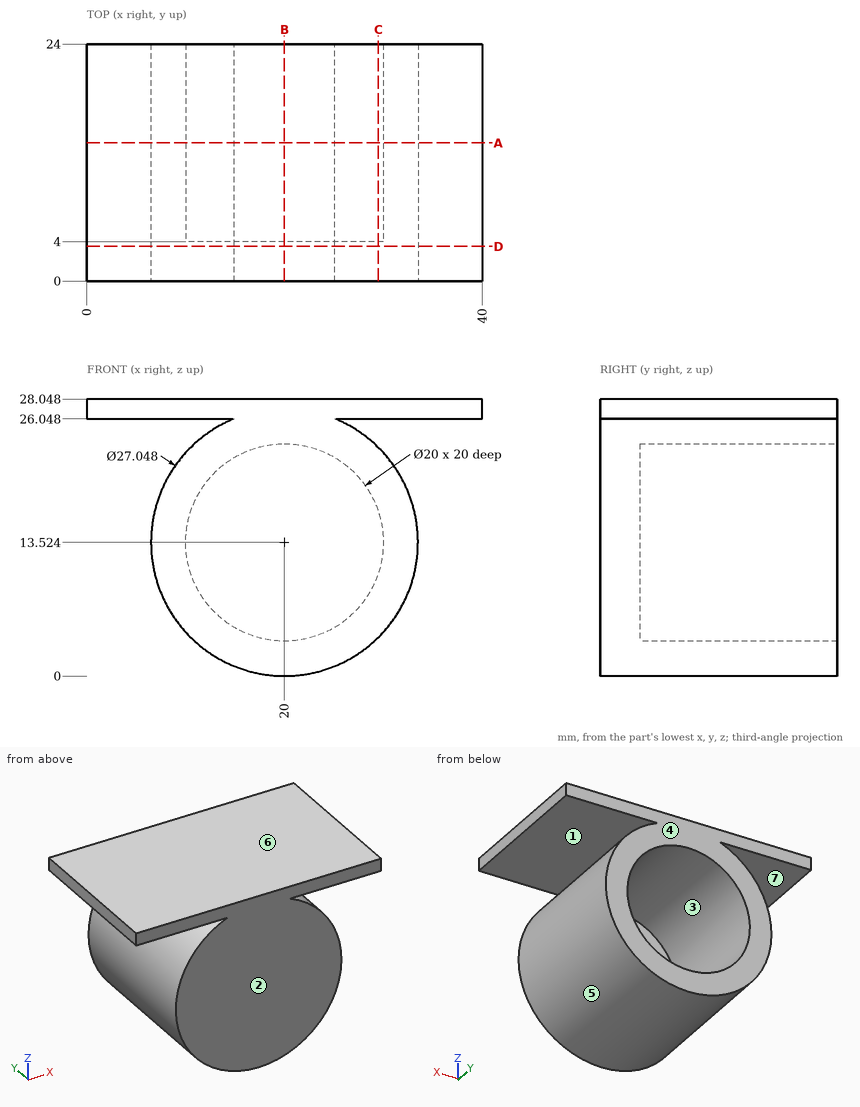
Geometry: see drawing. Coordinates: mm, zero at the bounding-box minimum. A direction names the side the tool comes from. Coordinates: 2 decimals unless noted, no trailing zeros. Loops run counter-clockwise (first coordinate to the right, second up) from the corner with the lowest first, then second, coordinate; pieces in that order, holes last. Notation, with made-up numbers: M 62,13 L 108,13 A8 ccw 108,20 Z; hole C 18.5,-20.5 d5. An arc over 180 degrees is marked long. Put each result on its own line as item: value. Start each with the question number.
1) Cut plane A-A on y = 14. Return the cut outline in (x, z), then the cut area to 3 significant figures.
2) Pull-direction query (Z, two-part tool) for the marked faces 4, 5, 6 and 7; classes: pulls with the +Z half, pulls with the -Z half, needs draft (parallel to the pull), parting line crosses it, or undercut.
3) Cut plane D-D on y = 3.5. Return the cut outline in (x, z), then the cut area to 3 significant figures.
4) Contact query for flat-ended pins moving along their axis: pin 1 Ø4 at (y, z) = (2.5, 7) entering from +X (3 decimals); pin 2 Ø4.5 at (x, y) = (11, 7) entering from -Z (3 decimals); pin 3 Ø6 at (x, y) = (7.5, 10) entering from -Z. Output: stop coordinate, or through.
5) Cut plane C-C on x = 29.5. Return the cut outline in (y, z).
6) Ray query, L1, parallel to Z at x = 29, y = 16.25 (1 decimal); L2, parallel to X at y = 12.25, z = 18.5 (1 decimal); L3, parallel to X at y = 6.25, z = 15.5. Return the intervals inside material, ascending. Write a range as from..to.
7) Cut plane B-B on x = 20. Return the cut outline in (y, z).
8) Reachability of the marked faces 1, 2 and 3 from +Z, -Z, +X, -X, +Y, -Y: full face, straight path, thin tool, end or side. Return the list, or none.
The answers:
1. outline: M 0,26.05 L 14.9,26.05 A13.52 ccw long 25.1,26.05 L 40,26.05 L 40,28.05 L 0,28.05 Z; hole C 20,13.52 d20
1. area: 334 mm²
2. face 4: needs draft
2. face 5: undercut
2. face 6: pulls with the +Z half
2. face 7: undercut
3. outline: M 0,26.05 L 14.9,26.05 A13.52 ccw long 25.1,26.05 L 40,26.05 L 40,28.05 L 0,28.05 Z
3. area: 648 mm²
4. pin 1: stops at x = 32.745
4. pin 2: stops at z = 1.805
4. pin 3: stops at z = 3.9
5. outline: M 0,3.9 L 24,3.9 L 24,10.4 L 4,10.4 L 4,16.65 L 24,16.65 L 24,23.15 L 0,23.15 Z; M 0,26.05 L 24,26.05 L 24,28.05 L 0,28.05 Z
6. L1: z = 3.4..9.2, 17.9..23.6, 26..28
6. L2: x = 7.4..11.3, 28.7..32.6
6. L3: x = 6.62..10.2, 29.8..33.38
7. outline: M 0,0 L 24,0 L 24,3.52 L 4,3.52 L 4,23.52 L 24,23.52 L 24,28.05 L 0,28.05 Z
8. face 1: +X, +Y, -Y
8. face 2: +Z, -Z, +X, -X, -Y
8. face 3: +Y
